For this review, take the finished solid that the model builds, in its own axes (mm). Give positions to 0.01 mm unless a question says otherwise; leave off trailing zeros. Loops run counter-clockwise (first coordinate to the right, second up) from the corner with the lowest first, then second, coordinate; pieces in that order, holes last. Notation, with made-up numbers: (39.25, -22.5) - (59.25, -22.5) arc R9 cw to (59.25, -10.5) - close; hole circle Ø10 at (6, 27.25). An arc over 180 degrees is marked (long way). Answer as CSV lines item,"result".
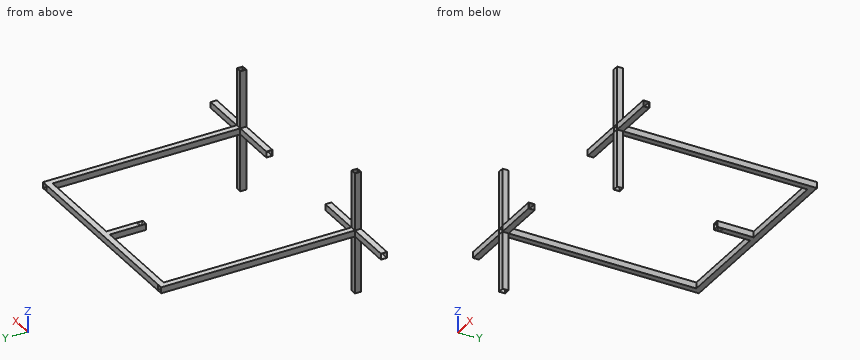
from build123d import *

# Parameters (mm, degrees)
SKETCH1_W           = 25
SKETCH1_H           = 25
SKETCH1_W_2         = 23
SKETCH1_H_2         = 23
BOSS_EXTRUDE1_DEPTH = 250
SKETCH2_W           = 25
SKETCH2_H           = 25
SKETCH2_W_2         = 23
SKETCH2_H_2         = 23
BOSS_EXTRUDE2_DEPTH = 200
SKETCH4_W           = 25
SKETCH4_H           = 25
CUT_EXTRUDE6_DEPTH  = 25
BOSS_EXTRUDE3_START = -12.5
SKETCH3_W           = 25
SKETCH3_H           = 25
SKETCH3_W_2         = 23
SKETCH3_H_2         = 23
BOSS_EXTRUDE3_DEPTH = 825
SKETCH5_W           = 25
SKETCH5_H           = 25
SKETCH5_W_2         = 23
SKETCH5_H_2         = 23
BOSS_EXTRUDE4_DEPTH = 400
SKETCH6_W           = 25
SKETCH6_H           = 25
SKETCH6_W_2         = 23
SKETCH6_H_2         = 23
BOSS_EXTRUDE5_DEPTH = 150
SKETCH7_R           = 2
CUT_EXTRUDE7_DEPTH  = 25


with BuildPart() as part:
    # Sketch1 → Boss-Extrude1 (new, symmetric)
    with BuildSketch(Plane.XY):
        Rectangle(SKETCH1_W, SKETCH1_H)
        Rectangle(SKETCH1_W_2, SKETCH1_H_2, mode=Mode.SUBTRACT)
    boss_extrude1 = extrude(amount=BOSS_EXTRUDE1_DEPTH, both=True)

    # Sketch2 → Boss-Extrude2 (add, symmetric)
    with BuildSketch(Plane(origin=(0, 0, 0), x_dir=(0, 0, -1), z_dir=(1, 0, 0))):
        Rectangle(SKETCH2_W, SKETCH2_H)
        Rectangle(SKETCH2_W_2, SKETCH2_H_2, mode=Mode.SUBTRACT)
    boss_extrude2 = extrude(amount=BOSS_EXTRUDE2_DEPTH, both=True)

    # Sketch4 → Cut-Extrude6 (cut)
    with BuildSketch(Plane.XZ.offset(12.5)):
        Rectangle(SKETCH4_W, SKETCH4_H)
    cut_extrude6 = extrude(amount=-CUT_EXTRUDE6_DEPTH, mode=Mode.SUBTRACT)


with BuildPart() as cut_extrude6_piece_1:
    # of the separate pieces the step leaves, piece 1, a body of its own (cut_extrude6_pieces)
    add(part.part.solids().sort_by_distance((-12.5, 12.5, -250))[0])



with BuildPart() as cut_extrude6_piece_2:
    # of the separate pieces the step leaves, piece 2, a body of its own (cut_extrude6_pieces)
    add(part.part.solids().sort_by_distance((-12.5, 12.5, 250))[0])


with BuildPart() as cut_extrude6_piece_3:
    # of the separate pieces the step leaves, piece 3, a body of its own (cut_extrude6_pieces)
    add(part.part.solids().sort_by_distance((-200, 12.5, -12.5))[0])


with BuildPart() as cut_extrude6_piece_4:
    # of the separate pieces the step leaves, piece 4, a body of its own (cut_extrude6_pieces)
    add(part.part.solids().sort_by_distance((200, 12.5, 12.5))[0])


with BuildPart() as cut_extrude6_piece_1_1:
    add(cut_extrude6_piece_1.part)

    add(cut_extrude6_piece_2.part)  # Boss-Extrude3 merges Cut-Extrude6 piece 2

    add(cut_extrude6_piece_3.part)  # Boss-Extrude3 merges Cut-Extrude6 piece 3

    add(cut_extrude6_piece_4.part)  # Boss-Extrude3 merges Cut-Extrude6 piece 4
    # Sketch3 → Boss-Extrude3 (add)
    with BuildSketch(Plane(origin=(0, 0, 0), x_dir=(1, 0, 0), z_dir=(0, 1, 0)).offset(BOSS_EXTRUDE3_START)):
        Rectangle(SKETCH3_W, SKETCH3_H)
        Rectangle(SKETCH3_W_2, SKETCH3_H_2, mode=Mode.SUBTRACT)
    boss_extrude3 = extrude(amount=BOSS_EXTRUDE3_DEPTH)

    # Sketch5 → Boss-Extrude4 (add)
    with BuildSketch(Plane.ZY.offset(12.5)):
        with Locations((0, 800)):
            Rectangle(SKETCH5_W, SKETCH5_H)
        with Locations((0, 800)):
            Rectangle(SKETCH5_W_2, SKETCH5_H_2, mode=Mode.SUBTRACT)
    boss_extrude4 = extrude(amount=BOSS_EXTRUDE4_DEPTH)

    # Mirror1: Boss-Extrude1, Boss-Extrude2, Cut-Extrude6, Boss-Extrude3, Boss-Extrude4 across plane
    add(boss_extrude1.mirror(Plane.ZY.offset(412.5)))
    add(boss_extrude2.mirror(Plane.ZY.offset(412.5)))
    add(cut_extrude6.mirror(Plane.ZY.offset(412.5)), mode=Mode.SUBTRACT)
    add(boss_extrude3.mirror(Plane.ZY.offset(412.5)))
    add(boss_extrude4.mirror(Plane.ZY.offset(412.5)))

    # Sketch6 → Boss-Extrude5 (add)
    with BuildSketch(Plane.XZ.offset(-787.5)):
        with Locations((-412.5, 0)):
            Rectangle(SKETCH6_W, SKETCH6_H)
        with Locations((-412.5, 0)):
            Rectangle(SKETCH6_W_2, SKETCH6_H_2, mode=Mode.SUBTRACT)
    extrude(amount=BOSS_EXTRUDE5_DEPTH)

    # Sketch7 → Cut-Extrude7 (cut)
    with BuildSketch(Plane.XY.offset(12.5)):
        with Locations((-420, 662.5)):
            Circle(SKETCH7_R)
        with Locations((-405, 662.5)):
            Circle(SKETCH7_R)
        with Locations((-420, 652.5)):
            Circle(SKETCH7_R)
        with Locations((-405, 652.5)):
            Circle(SKETCH7_R)
        with Locations((-420, 642.5)):
            Circle(SKETCH7_R)
        with Locations((-405, 642.5)):
            Circle(SKETCH7_R)
    extrude(amount=-CUT_EXTRUDE7_DEPTH, mode=Mode.SUBTRACT)


solid = cut_extrude6_piece_1_1.part
1) Insertion check: P1, Ø5, axis at x = -369.5, z = 16, coming from the -Y side; P2, Ø7.5, axis at x = 74.5, z = -6, coming from the +Y side; P3, Ø6, axis at y = 577.5, z = 5, coming from the +X side; P4, Ø6.5, axis at x = -405, y = 642.5, coming from the -Z side. Each pin has a flat end and moves straight along its axis. Give the tip position at first contact, or say it passes through.
From the geometry:
P1,"passes through"
P2,"stops at y = 12.5"
P3,"stops at x = 12.5"
P4,"stops at z = -12.5"
2) Consider section A-A on y = 216. Write out the cut boundary in (x, z).
From the geometry:
outline,"(-837.5, -12.5) - (-812.5, -12.5) - (-812.5, 12.5) - (-837.5, 12.5) - close; (-12.5, -12.5) - (12.5, -12.5) - (12.5, 12.5) - (-12.5, 12.5) - close; hole (-836.5, -11.5) - (-813.5, -11.5) - (-813.5, 11.5) - (-836.5, 11.5) - close; hole (-11.5, -11.5) - (11.5, -11.5) - (11.5, 11.5) - (-11.5, 11.5) - close"
3) Consider section C-C on x = -310. Write out the cut boundary in (y, z).
From the geometry:
outline,"(787.5, -12.5) - (812.5, -12.5) - (812.5, 12.5) - (787.5, 12.5) - close; hole (788.5, -11.5) - (811.5, -11.5) - (811.5, 11.5) - (788.5, 11.5) - close"
4) Wall thickness on line 1 (X direction, y = 652.5, z = -12.05); line 2 (Y direction, x = -420, z = -11); line 3 (Y direction, x = 3, z = 215.5): over which ranges is each line inside the solid? List them lowest first. Write a range as from..to.
From the geometry:
line 1,"x = -837.5..-812.5, -425..-422, -418..-407, -403..-400, -12.5..12.5"
line 2,"y = 787.5..788.5, 811.5..812.5"
line 3,"y = -12.5..-11.5, 11.5..12.5"
